Answer from the drawing. Dimensions are ordinates in mm from the lowest x, y and z of the part. A direction names the side the tool comes from. Coordinates: 2 decimals unless noted, no trailing zeros. Write each loop counter-clockwise with the first axis right and the second up, starting at its lowest first coordinate (ties: lowest second). Pieces come first, ordered by that corner, then holes.
1) Each of these flat-tipped pins is pushed along its axis until it touches: pin 1 Ø4 at (x, y) = (85.5, 7.5) entering from -Z; pin 2 Ø22.5 at (x, z) = (25.5, 29) entering from +Y; pin 3 Ø1.6 at (x, z) = (28.5, 43.5) entering from +Y. Where does it stop, or does it pass through?
2) The part is cut by section B-B (z = 44). Determine the outline of the cut face in (x, y), then the cut area to 3 significant figures.
3) The part is cut by section D-D (z = 26). Determine the outline of the cut face in (x, y).
4) Find the intervals of material crossed by line 1 (X direction, y = 19.75, z = 40); line 2 (Z direction, x = 5, y = 10); line 3 (Z direction, x = 56, y = 6.25), in increasing order.
5) The part is cut by section C-C (x = 8.5). Determine the outline of the cut face in (y, z).
6) Which of the six approach directions +Z, -Z, +X, -X, +Y, -Y give full straight-line access (tool end or side, diameter ignored) to the marked faces 1 and 2?
7) Determine the mould class of the marked faces 3, 4 and 5 for opening direction Z: +Z half, -Z half, draft (parallel to the pull), parting line (faces both ways), or undercut.
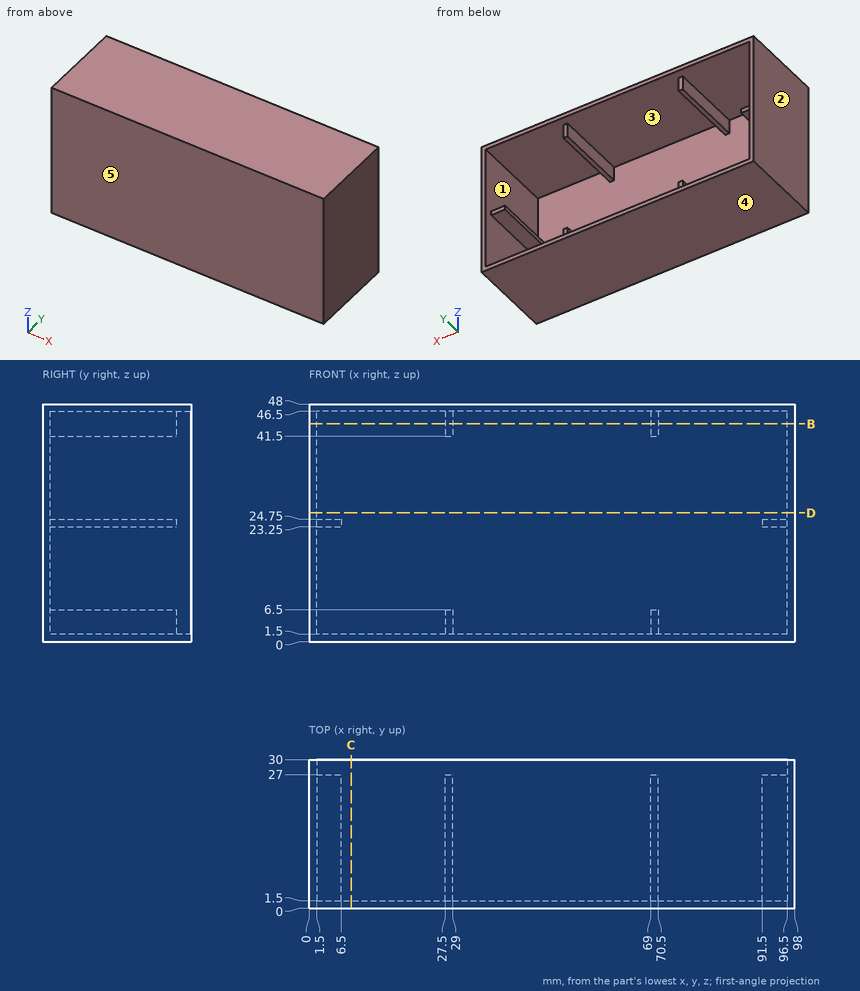
Reported:
1. pin 1: stops at z = 0
1. pin 2: stops at y = 1.5
1. pin 3: stops at y = 27
2. outline: (0, 0) - (98, 0) - (98, 30) - (96.5, 30) - (96.5, 1.5) - (70.5, 1.5) - (70.5, 27) - (69, 27) - (69, 1.5) - (29, 1.5) - (29, 27) - (27.5, 27) - (27.5, 1.5) - (1.5, 1.5) - (1.5, 30) - (0, 30) - close
2. area: 309 mm2
3. outline: (0, 0) - (98, 0) - (98, 30) - (96.5, 30) - (96.5, 1.5) - (1.5, 1.5) - (1.5, 30) - (0, 30) - close
4. line 1: x = 0 to 1.5, 96.5 to 98
4. line 2: z = 0 to 1.5, 23.25 to 24.75, 46.5 to 48
4. line 3: z = 0 to 1.5, 46.5 to 48
5. outline: (0, 0) - (30, 0) - (30, 1.5) - (1.5, 1.5) - (1.5, 46.5) - (30, 46.5) - (30, 48) - (0, 48) - close
6. face 1: +Y
6. face 2: +Z, -Z, -X, +Y, -Y
7. face 3: undercut
7. face 4: -Z half
7. face 5: draft
